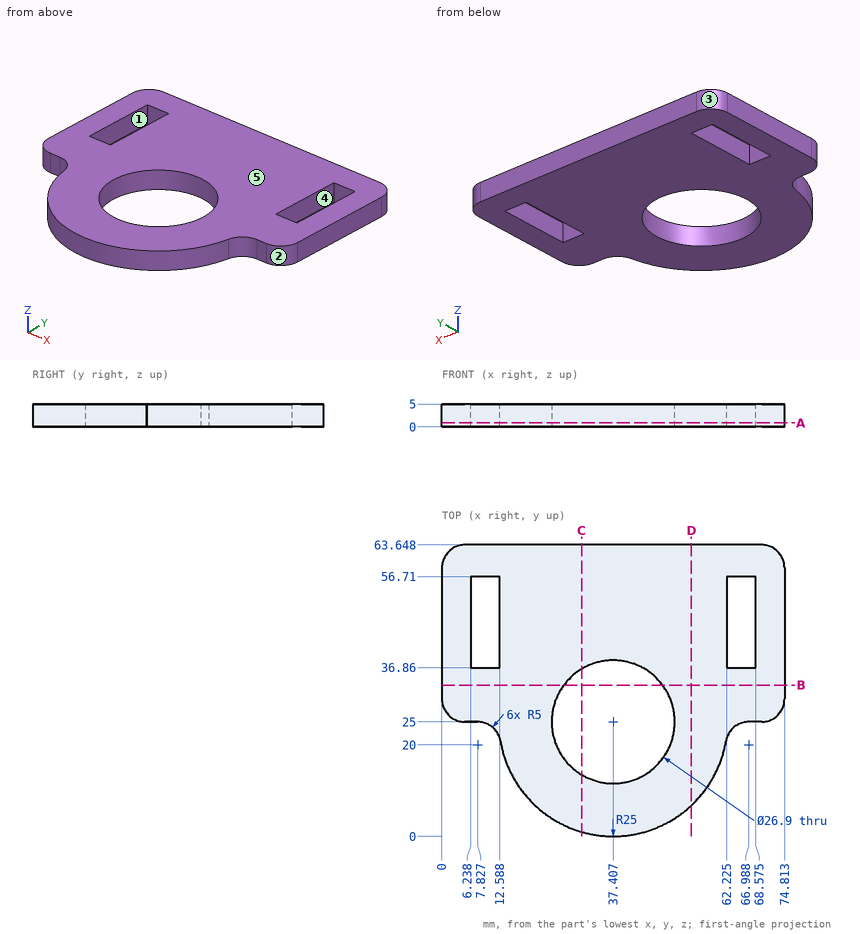
Check sheet for the drawn part. Datum: minimum x, y, z corner. Units: mm. A direction names the side the tool comes from. Round coordinates to 2 decimals unless told otherwise and drop trailing zeros. Write each loop counter-clockwise with the first axis right and the second up, starting at its lowest first coordinate (ties: lowest second). Pieces come first, ordered by that corner, then holes. Notation, with made-up numbers: (-24.5, 69.25) -> (-3.5, 69.25) arc R10 cw to (-3.5, 87.25) -> close; hole circle Ø4 at (14, 68.5). An arc over 180 degrees is marked (long way). Write each question's results on one line, items separated by ' | '. Start each with the question number.
1. Cross-section at D-D (x = 54.5). Enter the section's corners in (y, z).
2. Cross-section at B-B (y = 33). Enter the section's corners in (x, z) (1 decimal), then the cut area to 3 significant figures.
3. Material ranges on probe 1 along X at (y, z) = (46, 0.3) (1 decimal); probe 2 along X at (y, z) = (27, 0.85) (1 decimal); probe 3 along X at (y, z) = (59, 4.85), recorded low to high. Write a range as from..to.
4. Cross-section at C-C (x = 30.5). Enter the section's corners in (y, z), then the cut area to 3 significant figures.
5. Draft check along Y on the marked faces 3, 4 and 5. Enter one of: +Y half, -Y half, draft (parallel to the pull), parting line (faces both ways), or undercut.
6. Set-up check for the marked faces 1 and 2: record each of +Z, -Z, +X, -X, +Y, -Y from which the full face is reachable in a straight line by a thin tool's end or side.
7. Depth check by flat-ended pin: P1, Ø1.4, axis at x = 6.5, z = 3.5, coming from the -Y side; P2, Ø16, axis at x = 37.41, y = 25, coming from the +Z side (3 decimals); P3, Ø1.5, axis at x = 67, z = 3.5, coming from the -Y side (1 decimal). Enter the tip coordinate at first touch or a pass-through.
8. Cross-section at A-A (z = 0.9). Count the separate pieces of the cut face and the enclosed holes in it, then the cut area to 3 significant figures.
Solutions:
1) outline: (6.76, 0) -> (63.65, 0) -> (63.65, 5) -> (6.76, 5) -> close
2) outline: (0, 0) -> (26.6, 0) -> (26.6, 5) -> (0, 5) -> close; (48.2, 0) -> (74.8, 0) -> (74.8, 5) -> (48.2, 5) -> close | area: 266 mm2
3) probe 1: x = 0..6.2, 12.6..62.2, 68.6..74.8 | probe 2: x = 1..24.1, 50.7..73.8 | probe 3: x = 0.01..74.8
4) outline: (0.97, 0) -> (13.46, 0) -> (13.46, 5) -> (0.97, 5) -> close; (36.54, 0) -> (63.65, 0) -> (63.65, 5) -> (36.54, 5) -> close | area: 198 mm2
5) face 3: +Y half | face 4: undercut | face 5: draft
6) face 1: +Z, -Z | face 2: +Z, -Z, +X, -Y
7) P1: stops at y = 25 | P2: passes through | P3: stops at y = 24.9
8) separate pieces: 1 | enclosed holes: 3 | area: 3,040 mm2
